CAD build for the part. Positions are in the model's coordinates, mm. Round coordinates to 2 decimals unless told otherwise and drop trailing zeros. Write each loop counter-clockwise with the first axis right and the second up, starting at its lowest first coordinate (ties: lowest second). Pieces come first, ordered by that corner, then holes. Notation, with made-up numbers: (80.25, -31) - (138.25, -31) arc R30 ccw to (138.25, 3) - close; hole circle Ø7 at (-19, 62.5). An arc over 180 degrees is marked (long way). Answer in a Markdown table with one row per item.
```python
from build123d import *

# Parameters (mm, degrees)
SKETCH2_R           = 12.25
BOSS_EXTRUDE1_DEPTH = 5
CUT_EXTRUDE1_REACH  = 70.4
SKETCH3_R           = 1.5


with BuildPart() as part:
    # Sketch2 → Boss-Extrude1 (new body)
    # profile 1 of 6: a face of its own
    with BuildSketch(Plane(origin=(0, 0, 0), x_dir=(1, 0, 0), z_dir=(0, 1, 0))):
        with BuildLine():
            ThreePointArc((-37.10126952, 30.670072063), (-34.291787618, 30.469762498), (-31.819805153, 31.819805153))
            Line((-31.819805153, 31.819805153), (-38.890872965, 38.890872965))
            ThreePointArc((-38.890872965, 38.890872965), (-40.24091562, 34.291787618), (-37.10126952, 30.670072063))
        make_face()
    # profile 2 of 6: a face of its own
    with BuildSketch(Plane(origin=(0, 0, 0), x_dir=(1, 0, 0), z_dir=(0, 1, 0))):
        with BuildLine():
            Line((-38.890872965, 38.890872965), (-31.819805153, 31.819805153))
            ThreePointArc((-31.819805153, 31.819805153), (0, 45), (31.819805153, 31.819805153))
            ThreePointArc((31.819805153, 31.819805153), (34.291787618, 30.469762498), (37.10126952, 30.670072063))
            ThreePointArc((37.10126952, 30.670072063), (40.24091562, 34.291787618), (38.890872965, 38.890872965))
            ThreePointArc((38.890872965, 38.890872965), (0, 55), (-38.890872965, 38.890872965))
        make_face()
    # profile 3 of 6: a face of its own
    with BuildSketch(Plane(origin=(0, 0, 0), x_dir=(1, 0, 0), z_dir=(0, 1, 0))):
        with BuildLine():
            ThreePointArc((31.819805153, 31.819805153), (0, 45), (-31.819805153, 31.819805153))
            ThreePointArc((-31.819805153, 31.819805153), (-32.980620877, 30.615006885), (-34.095849533, 29.367891389))
            add(Edge.make_bspline(
                [(-34.095849533, 29.367891389), (-29.412092921, 27.041011889), (-19.283887533, 18.248514738), (-16.048568895, 5.169213632), (-14.472968185, -2.845292938)],
                knots=[0.074524007, 0.074524007, 0.074524007, 0.074524007, 0.434164212, 1, 1, 1, 1], degree=3))
            ThreePointArc((-14.472968185, -2.845292938), (-1.42937386, 14.68057868), (14.75, 0))
            ThreePointArc((14.75, 0), (14.68057868, -1.42937386), (14.472968185, -2.845292938))
            add(Edge.make_bspline(
                [(34.095849533, 29.367891389), (29.412092921, 27.041011889), (19.283887533, 18.248514738), (16.048568895, 5.169213632), (14.472968185, -2.845292938)],
                knots=[0.074524007, 0.074524007, 0.074524007, 0.074524007, 0.434164212, 1, 1, 1, 1], degree=3))
            ThreePointArc((34.095849533, 29.367891389), (32.980620877, 30.615006885), (31.819805153, 31.819805153))
        make_face()
    # profile 4 of 6: a face of its own
    with BuildSketch(Plane(origin=(0, 0, 0), x_dir=(1, 0, 0), z_dir=(0, 1, 0))):
        with BuildLine():
            ThreePointArc((-34.095849533, 29.367891389), (-32.980620877, 30.615006885), (-31.819805153, 31.819805153))
            ThreePointArc((-31.819805153, 31.819805153), (-34.291787618, 30.469762498), (-37.10126952, 30.670072063))
            add(Edge.make_bspline(
                [(-37.10126952, 30.670072063), (-36.069084867, 30.285436005), (-35.066409295, 29.850063244), (-34.095849533, 29.367891389)],
                knots=[0, 0, 0, 0, 0.074524007, 0.074524007, 0.074524007, 0.074524007], degree=3))
        make_face()
    # profile 5 of 6: a face of its own
    with BuildSketch(Plane(origin=(0, 0, 0), x_dir=(1, 0, 0), z_dir=(0, 1, 0))):
        with BuildLine():
            ThreePointArc((37.10126952, 30.670072063), (34.291787618, 30.469762498), (31.819805153, 31.819805153))
            ThreePointArc((31.819805153, 31.819805153), (32.980620877, 30.615006885), (34.095849533, 29.367891389))
            add(Edge.make_bspline(
                [(37.10126952, 30.670072063), (36.069084867, 30.285436005), (35.066409295, 29.850063244), (34.095849533, 29.367891389)],
                knots=[0, 0, 0, 0, 0.074524007, 0.074524007, 0.074524007, 0.074524007], degree=3))
        make_face()
    # profile 6 of 6: a face of its own
    with BuildSketch(Plane(origin=(0, 0, 0), x_dir=(1, 0, 0), z_dir=(0, 1, 0))):
        with BuildLine():
            ThreePointArc((14.75, 0), (-1.42937386, 14.68057868), (-14.472968185, -2.845292938))
            ThreePointArc((-14.472968185, -2.845292938), (0, -14.75), (14.472968185, -2.845292938))
            ThreePointArc((14.472968185, -2.845292938), (14.68057868, -1.42937386), (14.75, 0))
        make_face()
        with Locations(Location((0, 0, 0), (0, 0, 270))):
            Circle(SKETCH2_R, mode=Mode.SUBTRACT)
    extrude(amount=BOSS_EXTRUDE1_DEPTH)

    # Sketch3 → Cut-Extrude1 (cut, up to next)
    with BuildSketch(Plane(origin=(0, 5, 0), x_dir=(1, 0, 0), z_dir=(0, 1, 0)), mode=Mode.PRIVATE) as cut_extrude1_sk1:
        with Locations(Location((-35.355339059, 35.355339059, 0), (0, 0, 270))):
            Circle(SKETCH3_R)
    cut_extrude1_tool1 = extrude(cut_extrude1_sk1.sketch, amount=-CUT_EXTRUDE1_REACH, mode=Mode.PRIVATE) & part.part
    # Sketch3 → Cut-Extrude1 (cut, up to next)
    with BuildSketch(Plane(origin=(0, 5, 0), x_dir=(1, 0, 0), z_dir=(0, 1, 0)), mode=Mode.PRIVATE) as cut_extrude1_sk2:
        with Locations(Location((35.355339059, 35.355339059, 0), (0, 0, 270))):
            Circle(SKETCH3_R)
    cut_extrude1_tool2 = extrude(cut_extrude1_sk2.sketch, amount=-CUT_EXTRUDE1_REACH, mode=Mode.PRIVATE) & part.part
    add(cut_extrude1_tool1.solids().sort_by_distance((-35.355339, 5, -35.355339))[0], mode=Mode.SUBTRACT)
    add(cut_extrude1_tool2.solids().sort_by_distance((35.355339, 5, -35.355339))[0], mode=Mode.SUBTRACT)


solid = part.part
```
Q1. Pull direction Z, two halves, no side cores. Call faces 1 (the cylindrical face through (-40.255, 2.465, -34.36)), 2 (the cylindrical face through (-0.284, 2.465, 14.747)), 3 (the cylindrical face through (3.68, 2.465, 11.684)): released by +Z, released by -Z, zero draft, split by the parting line, or undercut.
Computed:
| item | result |
|---|---|
| face 1 | split by the parting line |
| face 2 | released by +Z |
| face 3 | undercut |
Q2. Drill centre lines: line 1 (Z direction, x = 4.5, y = 2.75); line 2 (Z direction, x = 9.5, y = 1.1); line 3 (X direction, y = 3.9, z = -44.5). Where is each one in solid material? Low to high.
Computed:
| item | result |
|---|---|
| line 1 | z = -54.82 to -11.39, 11.39 to 14.05 |
| line 2 | z = -54.17 to -7.73, 7.73 to 11.28 |
| line 3 | x = -32.32 to 32.32 |
Q3. Saw through at D-D on z = -47. List the corners of the cut face in (x, y).
Computed:
| item | result |
|---|---|
| outline | (-28.57, 0) - (28.57, 0) - (28.57, 5) - (-28.57, 5) - close |
Q4. Saw through at A-A on x = 0. List the corners of the cut face in (y, z), then the cut area to 3 significant figures.
Computed:
| item | result |
|---|---|
| outline | (0, -55) - (5, -55) - (5, -12.25) - (0, -12.25) - close; (0, 12.25) - (5, 12.25) - (5, 14.75) - (0, 14.75) - close |
| area | 226 mm2 |
Q5. Saw through at C-C on y = 1. Count the separate pieces of the cut face and the enclosed holes in it, then the cut area to 3 significant figures.
Computed:
| item | result |
|---|---|
| separate pieces | 1 |
| enclosed holes | 3 |
| area | 2,710 mm2 |
Q6. Flat gauge pins, fed straight in: pin 1 (2 mm diameter, centred on x = 5, y = 4, fed in from +Z); pin 2 (3 mm diameter, centred on y = 4.5, z = -3.5, fed in from -X); pin 3 (2 mm diameter, centred on x = -3.5, y = 1.5, fed in from -Z). Where does each tip first touch, or does it go through?
Computed:
| item | result |
|---|---|
| pin 1 | stops at z = 14.2 |
| pin 2 | stops at x = -16.24 |
| pin 3 | stops at z = -54.94 |
Q7. Saw through at B-B on x = -9. List the corners of the cut face in (y, z), then the cut area to 3 significant figures.
Computed:
| item | result |
|---|---|
| outline | (0, -54.26) - (5, -54.26) - (5, -8.31) - (0, -8.31) - close; (0, 8.31) - (5, 8.31) - (5, 11.69) - (0, 11.69) - close |
| area | 247 mm2 |
